Input: part model. Units: mm. Frame: model coordinates. Give positions to 0.01 mm unless a question says otherwise; leave off trailing zeros. Write each loop counter-clockwise with the first axis right and the second up, starting at its lowest first coordinate (ties: lowest second). Pieces come first, ordered by that corner, then holes. Notation, with made-up numbers: (82, -32) - (93, -32) arc R36 cw to (93, 7) - close; hole circle Ø6 at (70.25, -3). An arc over 180 degrees is marked (long way). Use a Markdown table: item, result. Add a question column.
1. Material intervals for probe 1 along X at (y, z) = (1.25, -1.65); probe 2 along Z at (x, y) = (53, -5.5); probe 3 along X at (y, z) = (10.5, -2.9), sorted ascending.
2. Section query A-A, the plane y = -1.5. Return loops of the section in (x, z), plus the area to 3 significant figures.
3. Pin query (flat end, axial travel): pin 1 (2.5 mm diameter, centred on y = 10.5, z = -2, fed in from -X); pin 2 (1 mm diameter, centred on x = 43, z = -4.5, fed in from -Y); pin 3 (1.5 mm diameter, centred on y = -5, z = -1, fed in from +X); pin 4 (5.5 mm diameter, centred on x = 7.07, y = 1.48, fed in from +Z). Return the tip coordinate at first contact, or that it passes through.
4. Section query D-D, the plane y = -6. Return loops of the section in (x, z), plus the area to 3 significant figures.
5. Section query C-C, the plane x = 64. Return loops of the section in (y, z), plus the area to 3 significant figures.
```python
from build123d import *

# Parameters (mm, degrees)
ESBO_O1_R                = 4.5
RESSALTO_EXTRUS_O1_DEPTH = 3
ESBO_O1_9_R              = 4
ESBO_O1_9_R_2            = 2
RESSALTO_EXTRUS_O2_DEPTH = 5.5


with BuildPart() as part:
    # Esbo_o1 → Ressalto-extrus_o1 (new body)
    with BuildSketch(Plane.XY):
        Polygon((7.074470574, -10.667826967), (58.928805727, -10.667826967), (58.928805727, -8.667826967), (68.928805727, -8.667826967), (68.928805727, -10.667826967), (76.928805727, -10.667826967), (76.928805727, -8.667826967), (74.928805727, -8.667826967), (74.928805727, -2.667826967), (76.928805727, -2.667826967), (76.928805727, 6.332173033), (74.928805727, 6.332173033), (74.928805727, 12.332173033), (76.928805727, 12.332173033), (76.928805727, 14.332173033), (-10.925529426, 14.332173033), (-10.925529426, 12.332173033), (-8.987091583, 12.332173033), (-8.987091583, 6.332173033), (-10.925529426, 6.332173033), (-10.925529426, -2.667826967), (-8.987091583, -2.667826967), (-8.987091583, -8.667826967), (-10.925529426, -8.667826967), (-10.925529426, -10.667826967), (-2.925529426, -10.667826967), (-2.925529426, -8.667826967), (7.074470574, -8.667826967), align=None)
        with Locations((7.074470574, 1.482173033)):
            Circle(ESBO_O1_R, mode=Mode.SUBTRACT)
    extrude(amount=-RESSALTO_EXTRUS_O1_DEPTH)

    # Esbo_o1_9 → Ressalto-extrus_o2 (add)
    with BuildSketch(Plane.XY):
        with Locations((24.354470574, 1.482173033)):
            Circle(ESBO_O1_9_R)
        with Locations((24.354470574, 1.482173033)):
            Circle(ESBO_O1_9_R_2, mode=Mode.SUBTRACT)
        with Locations((41.854470574, 1.482173033)):
            Circle(ESBO_O1_9_R)
        with Locations((41.854470574, 1.482173033)):
            Circle(ESBO_O1_9_R_2, mode=Mode.SUBTRACT)
    extrude(amount=-RESSALTO_EXTRUS_O2_DEPTH)


solid = part.part
```
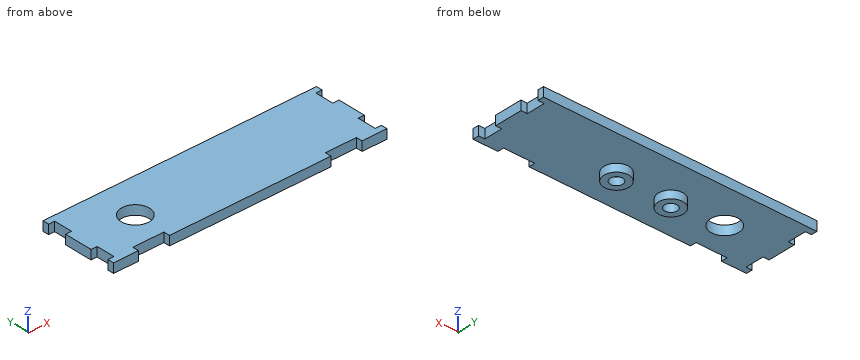
Result sheet:
| question | item | result |
|---|---|---|
| 1 | probe 1 | x = -10.93 to 2.58, 11.57 to 76.93 |
| 1 | probe 2 | z = -3 to 0 |
| 1 | probe 3 | x = -8.99 to 74.93 |
| 2 | outline | (-10.93, -3) - (3.7, -3) - (3.7, 0) - (-10.93, 0) - close; (10.44, -3) - (21.69, -3) - (21.69, -5.5) - (27.02, -5.5) - (27.02, -3) - (39.19, -3) - (39.19, -5.5) - (44.52, -5.5) - (44.52, -3) - (76.93, -3) - (76.93, 0) - (10.44, 0) - close |
| 2 | area | 270 mm² |
| 3 | pin 1 | stops at x = -8.99 |
| 3 | pin 2 | stops at y = -2.47 |
| 3 | pin 3 | stops at x = 74.93 |
| 3 | pin 4 | passes through |
| 4 | outline | (-8.99, -3) - (74.93, -3) - (74.93, 0) - (-8.99, 0) - close |
| 4 | area | 252 mm² |
| 5 | outline | (-8.67, -3) - (14.33, -3) - (14.33, 0) - (-8.67, 0) - close |
| 5 | area | 69.0 mm² |
